Read the model definition and answer for the solid it produces. Units are mm, in the model's axes. Face numbers are marked on the shaded views. A direction names the side the tool comes from. Give positions to 0.01 mm unless a question says otherwise; leave off trailing zeros. Loops run counter-clockwise (first coordinate to the right, second up) from the corner with the lowest first, then second, coordinate; pieces in that order, holes last.
(1) Find section C-C, the plane z = 39. Write down the section's boundary in (x, y), then the cut area to 3 significant figures.
(2) Which of the six approach directions +Z, -Z, +X, -X, +Y, -Y give full straight-line access (tool end or side, diameter ignored) to the marked faces 1, 2, 3 and 4?
(3) Find section B-B, the plane x = 0. Write down the section's boundary in (y, z), then the cut area to 3 significant figures.
(4) Straight lines are drawn through the part: probe 1 along Z at (x, y) = (0, -19); probe 2 along Z at (x, y) = (0, -24.4); probe 3 along Z at (x, y) = (26, -3). For each, find the intervals that lie inside material, in ascending order.
(5) Find section A-A, the plane z = 28.5. Write down the section's boundary in (x, y), then the cut area to 3 significant figures.
(6) Each of these flat-tipped pins is pushed along its axis until it touches: P1, Ø3, axis at x = 13.5, z = 32.5, coming from the +Y side; P2, Ø15, axis at x = -16.5, y = 5, coming from the +Z side; P3, Ø8, axis at y = -18, z = 21, coming from the -X side. Where does it stop, or does it pass through?
(7) Find section D-D, the plane x = -41. Write down the section's boundary in (y, z).
(8) Determine the mould class of the marked faces 5, 6 and 7 for opening direction X: pulls with the +X half, pulls with the -X half, needs draft (parallel to the pull), parting line crosses it, or undercut.
```python
from build123d import *

# Parameters (mm, degrees)
F0_W     = 114.3
F0_H     = 50.8
F1_DEPTH = 15.748
F2_R     = 15.875
F2_R_2   = 7.9375
F3_DEPTH = 15.748
F4_DEPTH = 3.048
F5_DEPTH = 50.801
F7_DEPTH = 15.749
F8_R     = 12.7


with BuildPart() as f1:
    # F0 (on Top) → F1 (new body)
    with BuildSketch(Plane.XY):
        Rectangle(F0_W, F0_H)
    extrude(amount=F1_DEPTH)

    # F2 (on face) → F3 (join)
    with BuildSketch(Plane.XZ.offset(25.4)):
        with BuildLine():
            Line((25.4, 15.748), (25.4, 34.798))
            ThreePointArc((25.4, 34.798), (0, 60.198), (-25.4, 34.798))
            Line((-25.4, 34.798), (-25.4, 15.748))
            Line((-25.4, 15.748), (25.4, 15.748))
        make_face()
        with Locations((0, 34.798)):
            Circle(F2_R, mode=Mode.SUBTRACT)
        with Locations((0, 34.798)):
            Circle(F2_R_2)
        with Locations((0, 34.798)):
            Circle(F2_R)
        with Locations((0, 34.798)):
            Circle(F2_R_2, mode=Mode.SUBTRACT)
    extrude(amount=-F3_DEPTH)

    # F2 (on face) → F4 (cut)
    with BuildSketch(Plane.XZ.offset(25.4)):
        with Locations((0, 34.798)):
            Circle(F2_R)
        with Locations((0, 34.798)):
            Circle(F2_R_2, mode=Mode.SUBTRACT)
    extrude(amount=-F4_DEPTH, mode=Mode.SUBTRACT)

    # F2 (on face) → F5 (cut, through all)
    with BuildSketch(Plane.XZ.offset(25.4)):
        with Locations((0, 34.798)):
            Circle(F2_R_2)
    extrude(amount=-F5_DEPTH, mode=Mode.SUBTRACT)

    # F6 (on face) → F7 (cut, through all)
    with BuildSketch(Plane.XY.offset(15.748)):
        with BuildLine():
            Line((-57.15, -4.826), (-44.45, -4.826))
            ThreePointArc((-44.45, -4.826), (-39.624, 0), (-44.45, 4.826))
            Line((-44.45, 4.826), (-57.15, 4.826))
            Line((-57.15, 4.826), (-57.15, -4.826))
        make_face()
        with BuildLine():
            Line((57.15, -4.826), (57.15, 4.826))
            Line((57.15, 4.826), (44.45, 4.826))
            ThreePointArc((44.45, 4.826), (39.624, 0), (44.45, -4.826))
            Line((44.45, -4.826), (57.15, -4.826))
        make_face()
    extrude(amount=-F7_DEPTH, mode=Mode.SUBTRACT)

    # F8
    f8_edges = [f1.edges().sort_by_distance(p)[0] for p in [
        (57.15, -25.4, 7.874),
        (57.15, 25.4, 7.874),
        (-57.15, -25.4, 7.874),
        (-57.15, 25.4, 7.874),
    ]]
    fillet(f8_edges, radius=F8_R)


solid = f1.part
```
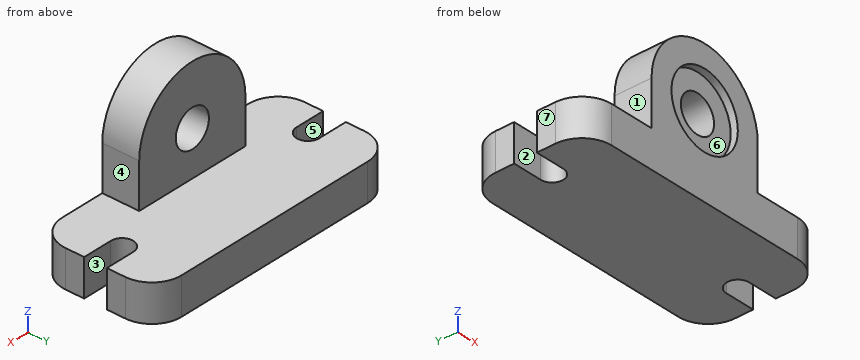
Entries:
1. outline: (-25.05, -25.4) - (-15.31, -25.4) - (-15.31, -22.35) - (-6.73, -22.35) - (-6.73, -9.65) - (-25.05, -9.65) - close; (6.73, -22.35) - (15.31, -22.35) - (15.31, -25.4) - (25.05, -25.4) - (25.05, -9.65) - (6.73, -9.65) - close
1. area: 525 mm2
2. face 1: +Z, -X, +Y, -Y
2. face 2: +Z, -Z, -X
2. face 3: +Z, -Z, +X
2. face 4: +Z, +X, +Y, -Y
3. outline: (-25.4, 0) - (25.4, 0) - (25.4, 15.75) - (-9.65, 15.75) - (-9.65, 26.86) - (-22.35, 26.86) - (-22.35, 18.92) - (-25.4, 18.92) - close; (-25.4, 50.67) - (-22.35, 50.67) - (-22.35, 42.74) - (-9.65, 42.74) - (-9.65, 60.2) - (-25.4, 60.2) - close
3. area: 1,200 mm2
4. probe 1: z = 0 to 26.86, 42.74 to 60.2
4. probe 2: z = 0 to 18.92, 50.67 to 60.2
4. probe 3: z = 0 to 15.75
5. outline: (-25.4, -25.4) - (-14.57, -25.4) - (-14.57, -22.35) - (-4.83, -22.35) - (-4.83, -9.65) - (-25.4, -9.65) - close; (4.83, -22.35) - (14.57, -22.35) - (14.57, -25.4) - (25.4, -25.4) - (25.4, -9.65) - (4.83, -9.65) - close
5. area: 588 mm2
6. P1: stops at y = -9.65
6. P2: stops at z = 15.75
6. P3: stops at x = -25.4
7. outline: (-25.4, 0) - (-3.37, 0) - (-3.37, 15.75) - (-25.4, 15.75) - close; (3.37, 0) - (25.4, 0) - (25.4, 15.75) - (3.37, 15.75) - close
8. face 5: needs draft
8. face 6: undercut
8. face 7: pulls with the -X half
